The listing builds one solid part. Answer for the finished solid, in the listing's coordinates (mm). Give positions to 0.01 mm unless a question says otherwise; leave off trailing zeros. Order: outer loops, then holes, each group sorted by start corner. A loop starts at its lowest first (then second) coordinate and runs counter-clockwise, first axis right, second up. Notation, with made-up numbers: (-1.5, -8) -> (44.5, -8) arc R21 ccw to (44.5, 15) -> close; hole circle Ø5 at (31, 57.25). An arc over 180 degrees is marked (long way). One line per question, with ' | ' between items. Start each with the question number.
```python
from build123d import *

# Parameters (mm, degrees)
CROQUIS1_W              = 10
CROQUIS1_H              = 3
SALIENTE_EXTRUIR1_DEPTH = 3
CROQUIS2_W              = 0.3
CROQUIS2_H              = 0.3
CROQUIS2_H_2            = 3
CORTAR_EXTRUIR2_DEPTH   = 3
CROQUIS3_W              = 3
CROQUIS3_H              = 3.5
CORTAR_EXTRUIR3_DEPTH   = 0.5
CROQUIS4_W              = 3
CROQUIS4_H              = 3.5
CORTAR_EXTRUIR4_DEPTH   = 0.5
CROQUIS5_W              = 3
CROQUIS5_H              = 3.5
CORTAR_EXTRUIR5_DEPTH   = 0.5
CROQUIS6_W              = 3
CROQUIS6_H              = 3.5
CORTAR_EXTRUIR6_DEPTH   = 0.5
REDONDEO1_START         = -1
REDONDEO1_DEPTH         = 5


with BuildPart() as part:
    # Croquis1 → Saliente-Extruir1 (new body)
    with BuildSketch(Plane.XY):
        with BuildLine():
            Line((-10, 70), (-10, 67))
            Line((-10, 67), (-7, 67))
            Line((-7, 67), (-7, 63))
            Line((-7, 63), (-9.5, 63))
            Line((-9.5, 63), (-9.5, 60))
            Line((-9.5, 60), (-0.5, 60))
            Line((-0.5, 60), (-0.5, 63))
            Line((-0.5, 63), (-3, 63))
            Line((-3, 63), (-3, 67))
            Line((-3, 67), (0, 67))
            Line((0, 67), (0, 70))
            Line((0, 70), (5, 70))
            Line((5, 70), (5, 67.405747627))
            ThreePointArc((5, 67.405747627), (4.929306729, 67.036438809), (4.727221995, 66.719345288))
            add(Edge.make_bspline(
                [(4.727221995, 66.719345288), (3.242407332, 65.146230192), (1.757592668, 62), (3.242407332, 58.853769808), (4.727221995, 57.280654712)],
                knots=[0.028065471, 0.028065471, 0.028065471, 0.028065471, 0.5, 0.971934529, 0.971934529, 0.971934529, 0.971934529], degree=3))
            ThreePointArc((4.727221995, 57.280654712), (4.929306729, 56.963561191), (5, 56.594252373))
            Line((5, 56.594252373), (5, 54.181314171))
            ThreePointArc((5, 54.181314171), (4.9841425, 54.003934523), (4.937072921, 53.832180471))
            add(Edge.make_bspline(
                [(4.937072921, 53.832180471), (3.31235764, 49.471453647), (1.68764236, 40.75), (3.31235764, 32.028546353), (4.937072921, 27.667819529)],
                knots=[0.006332812, 0.006332812, 0.006332812, 0.006332812, 0.5, 0.993667188, 0.993667188, 0.993667188, 0.993667188], degree=3))
            ThreePointArc((4.937072921, 27.667819529), (4.9841425, 27.496065477), (5, 27.318685829))
            Line((5, 27.318685829), (5, 24.567654138))
            ThreePointArc((5, 24.567654138), (4.997723384, 24.500214919), (4.990903903, 24.433082766))
            add(Edge.make_bspline(
                [(4.990903903, -48.933082766), (3.330301301, -36.70538851), (1.669698699, -12.25), (3.330301301, 12.20538851), (4.990903903, 24.433082766)],
                knots=[0.000910439, 0.000910439, 0.000910439, 0.000910439, 0.5, 0.999089561, 0.999089561, 0.999089561, 0.999089561], degree=3))
            ThreePointArc((4.990903903, -48.933082766), (4.997723384, -49.000214919), (5, -49.067654138))
            Line((5, -49.067654138), (5, -51.701381229))
            Line((5, -51.701381229), (5, -52))
            Line((5, -52), (0, -52))
            Line((0, -52), (0, -49))
            Line((0, -49), (-3, -49))
            Line((-3, -49), (-3, -45.5))
            Line((-3, -45.5), (-0.5, -45.5))
            Line((-0.5, -45.5), (-0.5, -42.5))
            Line((-0.5, -42.5), (-9.5, -42.5))
            Line((-9.5, -42.5), (-9.5, -45.5))
            Line((-9.5, -45.5), (-7, -45.5))
            Line((-7, -45.5), (-7, -49))
            Line((-7, -49), (-10, -49))
            Line((-10, -49), (-10, -52))
            Line((-10, -52), (-15, -52))
            Line((-15, -52), (-15, -51.701381229))
            Line((-15, -51.701381229), (-15, -49.067654138))
            ThreePointArc((-15, -49.067654138), (-14.997723384, -49.000214919), (-14.990903903, -48.933082766))
            add(Edge.make_bspline(
                [(-14.990903903, -48.933082766), (-13.330301301, -36.70538851), (-11.669698699, -12.25), (-13.330301301, 12.20538851), (-14.990903903, 24.433082766)],
                knots=[0.000910439, 0.000910439, 0.000910439, 0.000910439, 0.5, 0.999089561, 0.999089561, 0.999089561, 0.999089561], degree=3))
            ThreePointArc((-14.990903903, 24.433082766), (-14.997723384, 24.500214919), (-15, 24.567654138))
            Line((-15, 24.567654138), (-15, 27.318685829))
            ThreePointArc((-15, 27.318685829), (-14.9841425, 27.496065477), (-14.937072921, 27.667819529))
            add(Edge.make_bspline(
                [(-14.937072921, 53.832180471), (-13.31235764, 49.471453647), (-11.68764236, 40.75), (-13.31235764, 32.028546353), (-14.937072921, 27.667819529)],
                knots=[0.006332812, 0.006332812, 0.006332812, 0.006332812, 0.5, 0.993667188, 0.993667188, 0.993667188, 0.993667188], degree=3))
            ThreePointArc((-14.937072921, 53.832180471), (-14.9841425, 54.003934523), (-15, 54.181314171))
            Line((-15, 54.181314171), (-15, 56.594252373))
            ThreePointArc((-15, 56.594252373), (-14.929306729, 56.963561191), (-14.727221995, 57.280654712))
            add(Edge.make_bspline(
                [(-14.727221995, 57.280654712), (-13.242407332, 58.853769808), (-11.757592668, 62), (-13.242407332, 65.146230192), (-14.727221995, 66.719345288)],
                knots=[0.028065471, 0.028065471, 0.028065471, 0.028065471, 0.5, 0.971934529, 0.971934529, 0.971934529, 0.971934529], degree=3))
            ThreePointArc((-14.727221995, 66.719345288), (-14.929306729, 67.036438809), (-15, 67.405747627))
            Line((-15, 67.405747627), (-15, 70))
            Line((-15, 70), (-10, 70))
        make_face()
        with Locations((-5, 26)):
            Rectangle(CROQUIS1_W, CROQUIS1_H, mode=Mode.SUBTRACT)
        with Locations((-5, 55.5)):
            Rectangle(CROQUIS1_W, CROQUIS1_H, mode=Mode.SUBTRACT)
    extrude(amount=SALIENTE_EXTRUIR1_DEPTH)

    # Croquis2 → Cortar-Extruir2 (cut)
    with BuildSketch(Plane.XY.offset(3)):
        Polygon((-9.8, -45.5), (-9.8, -45.8), (-9.5, -45.8), (-7, -45.8), (-7, -45.5), (-9.5, -45.5), (-9.5, -42.5), (-0.5, -42.5), (-0.5, -42.2), (-9.5, -42.2), (-9.8, -42.2), (-9.8, -42.5), align=None)
        Polygon((-0.5, -45.8), (-0.2, -45.8), (-0.2, -45.5), (-0.2, -42.5), (-0.5, -42.5), (-0.5, -45.5), (-3, -45.5), (-3, -45.8), align=None)
        with Locations((-0.35, -42.35)):
            Rectangle(CROQUIS2_W, CROQUIS2_H)
        with Locations((-10.15, 26)):
            Rectangle(CROQUIS2_W, CROQUIS2_H_2)
        with Locations((0.15, 26)):
            Rectangle(CROQUIS2_W, CROQUIS2_H_2)
        with Locations((0.15, 55.5)):
            Rectangle(CROQUIS2_W, CROQUIS2_H_2)
        with Locations((-10.15, 55.5)):
            Rectangle(CROQUIS2_W, CROQUIS2_H_2)
        Polygon((-9.8, 63.3), (-9.5, 63.3), (-7, 63.3), (-7, 63), (-9.5, 63), (-9.5, 60), (-0.5, 60), (-0.5, 63), (-3, 63), (-3, 63.3), (-0.5, 63.3), (-0.2, 63.3), (-0.2, 63), (-0.2, 60), (-0.2, 59.7), (-0.5, 59.7), (-9.5, 59.7), (-9.8, 59.7), (-9.8, 60), (-9.8, 63), align=None)
    extrude(amount=-CORTAR_EXTRUIR2_DEPTH, mode=Mode.SUBTRACT)

    # Croquis3 → Cortar-Extruir3 (cut)
    with BuildSketch(Plane.ZY.offset(15)):
        with Locations((1.5, -50.25)):
            Rectangle(CROQUIS3_W, CROQUIS3_H)
    extrude(amount=-CORTAR_EXTRUIR3_DEPTH, mode=Mode.SUBTRACT)

    # Croquis4 → Cortar-Extruir4 (cut)
    with BuildSketch(Plane(origin=(5, 0, 0), x_dir=(0, 0, -1), z_dir=(1, 0, 0))):
        with Locations((-1.5, -50.25)):
            Rectangle(CROQUIS4_W, CROQUIS4_H)
    extrude(amount=-CORTAR_EXTRUIR4_DEPTH, mode=Mode.SUBTRACT)

    # Croquis5 → Cortar-Extruir5 (cut)
    with BuildSketch(Plane.ZY.offset(15)):
        with Locations((1.5, 68.25)):
            Rectangle(CROQUIS5_W, CROQUIS5_H)
    extrude(amount=-CORTAR_EXTRUIR5_DEPTH, mode=Mode.SUBTRACT)

    # Croquis6 → Cortar-Extruir6 (cut)
    with BuildSketch(Plane(origin=(5, 0, 0), x_dir=(0, 0, -1), z_dir=(1, 0, 0))):
        with Locations((-1.5, 68.25)):
            Rectangle(CROQUIS6_W, CROQUIS6_H)
    extrude(amount=-CORTAR_EXTRUIR6_DEPTH, mode=Mode.SUBTRACT)

    # Redondeo1: read off the stored shape, not the designer's step
    # Redondeo1 outline → Redondeo1 (cut)
    with BuildSketch(Plane.XY.offset(REDONDEO1_START)):
        with BuildLine():
            Line((-14.932435559, -48.5), (-14.5, -48.5))
            ThreePointArc((-14.5, -48.5), (-14.379883961, -45.021273255), (-14.08941772, -41.552614006))
            add(Edge.make_bspline(
                [(-14.932435559, -48.5), (-14.621648088, -46.184204669), (-14.340642142, -43.868409337), (-14.08941772, -41.552614006)],
                knots=[0.006802721, 0.006802721, 0.006802721, 0.006802721, 0.10132498, 0.10132498, 0.10132498, 0.10132498], degree=3))
        make_face()
        with BuildLine():
            add(Edge.make_bspline(
                [(4.932435559, -48.5), (4.621648088, -46.184204669), (4.340642142, -43.868409337), (4.08941772, -41.552614006)],
                knots=[0.006802721, 0.006802721, 0.006802721, 0.006802721, 0.10132498, 0.10132498, 0.10132498, 0.10132498], degree=3))
            ThreePointArc((4.08941772, -41.552614006), (4.379883961, -45.021273255), (4.5, -48.5))
            Line((4.5, -48.5), (4.932435559, -48.5))
        make_face()
        with BuildLine():
            Line((4.525, 66.5), (4.5, 66.5))
            ThreePointArc((4.5, 66.5), (4.313911858, 66.266314057), (4.126842149, 66.033413132))
            add(Edge.make_bspline(
                [(4.525, 66.5), (4.38502394, 66.344471044), (4.252304656, 66.188942088), (4.126842149, 66.033413132)],
                knots=[0.05, 0.05, 0.05, 0.05, 0.096658687, 0.096658687, 0.096658687, 0.096658687], degree=3))
        make_face()
        with BuildLine():
            add(Edge.make_bspline(
                [(-14.126842149, 66.033413132), (-14.252304656, 66.188942088), (-14.38502394, 66.344471044), (-14.525, 66.5)],
                knots=[0.903341313, 0.903341313, 0.903341313, 0.903341313, 0.95, 0.95, 0.95, 0.95], degree=3))
            ThreePointArc((-14.126842149, 66.033413132), (-14.313911858, 66.266314057), (-14.5, 66.5))
            Line((-14.5, 66.5), (-14.525, 66.5))
        make_face()
    extrude(amount=REDONDEO1_DEPTH, mode=Mode.SUBTRACT)


solid = part.part
```
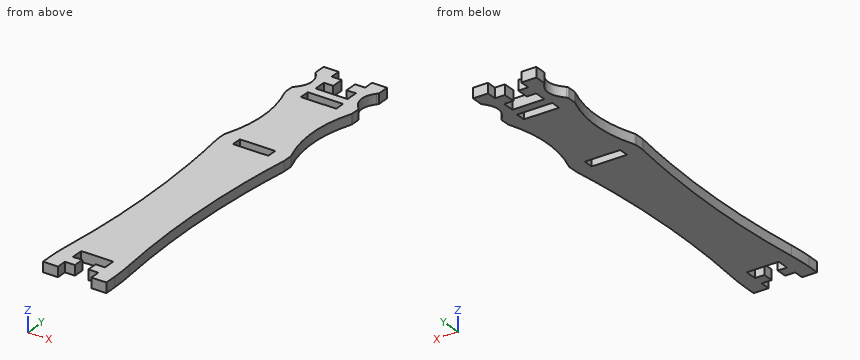
(1) The part is cut by section B-B on z = 0.5. State how many separate pieces and enclosed holes the cut face has, plus the area to 3 significant figures.
(2) Given P1, Ø1.5, axis at y = 67.5, z = 1.5, coming from the -X side; P2, Ø1.4, axis at x = -9, z = 2, coming from the +Y side, each flat-ended and moving along its own axis, determine where each tip first touches the part or whether it passes through.
(3) The part is cut by section A-A on x = -5. Determine the outline of the cut face in (y, z), plus the area to 3 significant figures.
(4) Consider line 1 (Y direction, x = -9.25, z = 1.8); line 2 (X direction, y = 27, z = 2); line 3 (X direction, y = 20.5, z = 1.45). Determine where each line is inside the solid, lowest interval first.
Result sheet:
1) separate pieces: 1 | enclosed holes: 2 | area: 1,840 mm^2
2) P1: stops at x = -14.5 | P2: stops at y = 67
3) outline: (-42.2, 0) -> (24.5, 0) -> (24.5, 3) -> (-42.2, 3) -> close; (27.5, 0) -> (54, 0) -> (54, 3) -> (27.5, 3) -> close; (57, 0) -> (59.7, 0) -> (59.7, 3) -> (57, 3) -> close | area: 288 mm^2
4) line 1: y = -49 to -45.8, -42.2 to 24.5, 27.5 to 54, 57 to 59.7, 63.3 to 67 | line 2: x = -15 to -10.3, 0.3 to 5 | line 3: x = -14.49 to 4.49
